```python
from build123d import *

# Parameters (mm, degrees)
SKETCH_1_W          = 40
SKETCH_1_H          = 95
SKETCH_1_R          = 4
SKETCH_1_R_2        = 1.6
EXTRUDE_1_DEPTH     = 6
SKETCH_2_W          = 40
SKETCH_2_H          = 5
EXTRUDE_2_DEPTH     = 14
SKETCH_3_R          = 6
CUT_EXTRUDE_1_DEPTH = 14
CHAMFER_1_SIZE      = 7
SKETCH_4_R          = 1.6
CUT_EXTRUDE_2_DEPTH = 14
FILLET_1_R          = 5
EXTRUDE_3_DEPTH     = 40
SKETCH_7_R          = 1.6
CUT_EXTRUDE_3_DEPTH = 40


with BuildPart() as part:
    # Эскиз1 → Бобышка-Вытянуть1 (new body)
    with BuildSketch(Plane(origin=(0, 0, 0), x_dir=(1, 0, 0), z_dir=(0, 1, 0))):
        with Locations((0, 47.5)):
            Rectangle(SKETCH_1_W, SKETCH_1_H)
        with Locations((0, 78)):
            Circle(SKETCH_1_R, mode=Mode.SUBTRACT)
        with Locations((-9, 87)):
            Circle(SKETCH_1_R_2, mode=Mode.SUBTRACT)
        with Locations((9, 87)):
            Circle(SKETCH_1_R_2, mode=Mode.SUBTRACT)
        with Locations((-9, 54)):
            Circle(SKETCH_1_R_2, mode=Mode.SUBTRACT)
        with Locations((9, 54)):
            Circle(SKETCH_1_R_2, mode=Mode.SUBTRACT)
    extrude(amount=EXTRUDE_1_DEPTH)

    # Эскиз2 → Бобышка-Вытянуть2 (add)
    with BuildSketch(Plane(origin=(0, 6, 0), x_dir=(1, 0, 0), z_dir=(0, 1, 0))):
        with Locations((0, 2.5)):
            Rectangle(SKETCH_2_W, SKETCH_2_H)
    extrude(amount=EXTRUDE_2_DEPTH)

    # Эскиз3 → Вырез-Вытянуть1 (cut)
    with BuildSketch(Plane(origin=(0, 0, -5), x_dir=(-1, 0, 0), z_dir=(0, 0, -1))):
        with Locations((0, 20)):
            Circle(SKETCH_3_R)
    extrude(amount=-CUT_EXTRUDE_1_DEPTH, mode=Mode.SUBTRACT)

    # Фаска1
    chamfer_1_edges = [part.edges().sort_by_distance(p)[0] for p in [
        (0, 6, -5),
    ]]
    chamfer(chamfer_1_edges, length=CHAMFER_1_SIZE)

    # Эскиз4 → Вырез-Вытянуть2 (cut)
    with BuildSketch(Plane(origin=(0, 0, -5), x_dir=(-1, 0, 0), z_dir=(0, 0, -1))):
        with Locations((13.5, 16.5)):
            Circle(SKETCH_4_R)
        with Locations((-13.5, 16.5)):
            Circle(SKETCH_4_R)
    extrude(amount=-CUT_EXTRUDE_2_DEPTH, mode=Mode.SUBTRACT)

    # Скругление1
    fillet_1_edges = [part.edges().sort_by_distance(p)[0] for p in [
        (-20, 3, -95),
        (20, 3, -95),
    ]]
    fillet(fillet_1_edges, radius=FILLET_1_R)

    # Эскиз5 → Бобышка-Вытянуть3 (add)
    with BuildSketch(Plane(origin=(20, 0, 0), x_dir=(0, 0, -1), z_dir=(1, 0, 0))):
        Polygon((5, -7), (5, -14), (0, -14), (0, 0), (12, 0), align=None)
    extrude(amount=-EXTRUDE_3_DEPTH)

    # Эскиз7 → Вырез-Вытянуть3 (cut)
    with BuildSketch(Plane.XY):
        with Locations((13.5, -10.5)):
            Circle(SKETCH_7_R)
        with Locations((-13.5, -10.5)):
            Circle(SKETCH_7_R)
    extrude(amount=-CUT_EXTRUDE_3_DEPTH, mode=Mode.SUBTRACT)


solid = part.part
```
Work out the finished part from the listing and answer in its coordinate system (mm). A direction names the side the tool comes from. Coordinates: 2 decimals unless noted, no trailing zeros. Loops run counter-clockwise (first coordinate to the right, second up) from the corner with the lowest first, then second, coordinate; pieces in that order, holes last.
1) Section A-A (x = 9) is taken. Give the vertices of the cut face in (y, z), plus the area to 3 significant figures.
Results:
outline: (-14, -5) - (-7, -5) - (0, -12) - (0, -52.4) - (6, -52.4) - (6, -12) - (13, -5) - (20, -5) - (20, 0) - (-14, 0) - close; (0, -95) - (6, -95) - (6, -88.6) - (0, -88.6) - close; (0, -85.4) - (6, -85.4) - (6, -55.6) - (0, -55.6) - close
area: 721 mm2
2) Section D-D (x = 0) is taken. Give the vertices of the cut face in (y, z).
Results:
outline: (-14, -5) - (-7, -5) - (0, -12) - (0, -74) - (6, -74) - (6, -12) - (13, -5) - (14, -5) - (14, 0) - (-14, 0) - close; (0, -95) - (6, -95) - (6, -82) - (0, -82) - close
3) Section C-C (y = -10.5) is taken. Give the vertices of the cut face in (x, z), plus the area to 3 significant figures.
Results:
outline: (-20, -5) - (-15.1, -5) - (-15.1, 0) - (-20, 0) - close; (-11.9, -5) - (11.9, -5) - (11.9, 0) - (-11.9, 0) - close; (15.1, -5) - (20, -5) - (20, 0) - (15.1, 0) - close
area: 168 mm2
4) For a pull along X with two mould halves and no side action, classify faces 1 (the cylindrical face through (-14.77, -11.47, -2.46)), 2 (the cylindrical face through (-12.32, 17.58, -2.54)), 3 (the flat face through (-20, 2, -35)), 4 (the flat face through (0, -3, -9)) as +X half, -X half, draft (parallel to the pull), parting line (faces both ways), or undercut.
Results:
face 1: undercut
face 2: undercut
face 3: -X half
face 4: draft
5) Consider probe 1 along Z at (x, y) = (-9, 3.45); probe 2 along Y at (x, z) = (13.5, -2.5); probe 3 along X at (y, z) = (3, -54). Determine where each line is inside the solid, lowest interval first.
Results:
probe 1: z = -95 to -88.6, -85.4 to -55.6, -52.4 to 0
probe 2: y = -14 to -12.1, -8.9 to 14.9, 18.1 to 20
probe 3: x = -20 to -10.6, -7.4 to 7.4, 10.6 to 20
6) For faces 5 (the flat face through (-0.3, 13.3, -5)), 6 (the flat face through (0, -10, -5)), 7 (the cylindrical face through (18, 3, -94)), determine the directions among +Z, -Z, +X, -X, +Y, -Y from which every point of the face is accessible in a straight line to the end or side of a thin tool.
Results:
face 5: -Z, +X, -X, +Y
face 6: -Z, +X, -X, -Y
face 7: -Z, +X, +Y, -Y
7) Section B-B (z = -78) is taken. Give the vertices of the cut face in (x, y).
Results:
outline: (-20, 0) - (-4, 0) - (-4, 6) - (-20, 6) - close; (4, 0) - (20, 0) - (20, 6) - (4, 6) - close
8) Flat-ended cylindrical pins translate along their axes: pin 1 (1.5 mm diameter, centred on x = -9.5, z = -46.5, fed in from +Y); pin 2 (7.5 mm diameter, centred on x = 2, y = -11, fed in from -Z); pin 3 (1 mm diameter, centred on x = 3, z = -32.5, fed in from -Y). Find the tip coordinate at first contact, or state that the pin passes through.
Results:
pin 1: stops at y = 6
pin 2: stops at z = -5
pin 3: stops at y = 0
